Autodesk Fusion 360 part; units mm, degrees
sketch "Sketch1" plane through (0, 0, 0) normal (0, 0, 1) x (1, 0, 0)
  circle A0 centre (0, 0) radius 44.45
  arc A1 (38.1661, 38.1661) -> (-38.1661, 38.1661) centre (0, 0) ccw
  line L0 (0, 0) -> (38.1661, 38.1661) construction
  line L1 (0, 0) -> (-38.1661, 38.1661) construction
  line L2 (-38.1661, 38.1661) -> (-31.4309, 31.4309) construction
  line L3 (-38.1661, 38.1661) -> (-31.4309, 31.4309)
  line L4 (31.4309, 31.4309) -> (38.1661, 38.1661)
  line L5 (0, 0) -> (0, 53.975) construction
  line L6 (0, 53.975) -> (-31.4309, 31.4309) construction
  line L7 (0, 53.975) -> (31.4309, 31.4309) construction
  line L8 (-13.335, 80.645) -> (13.335, 80.645)
  line L9 (13.335, 80.645) -> (13.335, 53.975)
  line L10 (13.335, 53.975) -> (-13.335, 53.975) construction
  line L11 (-13.335, 53.975) -> (-13.335, 80.645)
  line L12 (-13.335, 53.975) -> (-13.335, 52.3018)
  line L13 (13.335, 53.975) -> (13.335, 52.3018)
  line L14 (-13.335, 67.31) -> (13.335, 67.31) construction
  circle A2 centre (0, 67.31) radius 11.049
  point P0 (-31.4309, 31.4309)
  point P1 (-13.335, 52.3018)
  point P2 (13.335, 52.3018)
  point P3 (-13.335, 67.31)
  point P4 (13.335, 67.31)
  dimension "d1" = 88.9
  dimension "d2" = 90
  dimension "d3" = 9.525
  dimension "d6" = 26.67
  dimension "d7" = 26.67
  dimension "d8" = 22.098
extrude "Extrude2" add sketch "Sketch1" along normal blind 50.8 contours A0 A1 L3 L4 | A1 L8 L9 L11 L12 L13
fillet "Fillet1" radius 5 2 edges at (-38.1661, 38.1661, 25.4) (38.1661, 38.1661, 25.4)
fillet "Fillet2" radius 15 2 edges at (-13.335, 52.3018, 25.4) (13.335, 52.3018, 25.4)
fillet "Fillet3" radius 5 2 edges at (-13.335, 80.645, 25.4) (13.335, 80.645, 25.4)
sketch "Sketch4" plane through (0, 80.645, 0) normal (0, 1, 0) x (-1, 0, 0)
  line L0 (-8.335, 50.8) -> (-8.335, 0)
  line L1 (-8.335, 0) -> (8.335, 0)
  line L2 (8.335, 0) -> (8.335, 50.8)
  line L3 (8.335, 50.8) -> (-8.335, 50.8)
  line L4 (0, 0) -> (0, 16.9333) construction
  line L5 (0, 16.9333) -> (0, 33.8667) construction
  line L6 (0, 33.8667) -> (0, 50.8) construction
  circle A0 centre (0, 16.9333) radius 1.778
  circle A1 centre (0, 33.8667) radius 1.778
  dimension "d17" = 3.556
  dimension "d18" = 3.556
extrude "Extrude3" cut sketch "Sketch4" along normal up to surface contours A0 | A1 end surface at (10.9941, 66.2099, 33.8667)
sketch "Sketch6" plane through (0, 0, 50.8) normal (0, 0, 1) x (-1, 0, 0)
  arc A0 (-13.335, -75.645) -> (-8.335, -80.645) centre (-8.335, -75.645) ccw
  line L0 (-8.335, -80.645) -> (8.335, -80.645)
  arc A1 (8.335, -80.645) -> (13.335, -75.645) centre (8.335, -75.645) ccw
  line L1 (13.335, -75.645) -> (13.335, -62.8862)
  arc A2 (22.173, -49.2104) -> (13.335, -62.8862) centre (28.335, -62.8862) ccw
  arc A3 (22.173, -49.2104) -> (34.0702, -41.8632) centre (0, 0) ccw
  arc A4 (34.0702, -41.8632) -> (34.4496, -34.4496) centre (30.9141, -37.9851) ccw
  line L2 (34.4496, -34.4496) -> (31.4309, -31.4309)
  arc A5 (-31.4309, -31.4309) -> (31.4309, -31.4309) centre (0, 0) ccw
  line L3 (-31.4309, -31.4309) -> (-34.4496, -34.4496)
  arc A6 (-34.4496, -34.4496) -> (-34.0702, -41.8632) centre (-30.9141, -37.9851) ccw
  arc A7 (-34.0702, -41.8632) -> (-22.173, -49.2104) centre (0, 0) ccw
  arc A8 (-13.335, -62.8862) -> (-22.173, -49.2104) centre (-28.335, -62.8862) ccw
  line L4 (-13.335, -62.8862) -> (-13.335, -75.645)
  circle A9 centre (0, -67.31) radius 11.049
  line L5 (0, -56.261) -> (0, -44.45)
  circle A10 centre (0, -67.31) radius 11.049
  circle A11 centre (0, 0) radius 44.45
  line L6 (0.25, -56.261) -> (-0.25, -56.261)
  line L7 (-0.25, -56.261) -> (-0.25, -44.45)
  line L8 (-0.25, -44.45) -> (0.25, -44.45)
  line L9 (0.25, -44.45) -> (0.25, -56.261)
  line L10 (0, 0) -> (0, -53.975)
  dimension "d22" = 0.5
extrude "Extrude4" cut sketch "Sketch6" against normal blind 0.5 contours A5 L5 A11 L6 L7 L8 L10 | A5 L5 A11 L6 L8 L9 L10
Could you check a few things on this model? Use its own coordinates, in mm. A direction names the side the tool comes from. Give positions to 0.01 mm unless a question says otherwise; leave off trailing zeros. Loops run counter-clockwise (first coordinate to the right, second up) from the corner with the lowest first, then second, coordinate; pieces in that order, holes last. Notation, with made-up numbers: (87.5, 19.25) -> (145.5, 19.25) arc R12 ccw to (145.5, 30.25) -> close; hole circle Ø5 at (-21, 46). An arc over 180 degrees is marked (long way). Return JSON: item names as keys, results as strings.
Item 1: If we section it at B-B on z = 28.5: List the corners of the cut face in (x, y) for me (3 decimals), plus the area to 3 significant figures.
Geometry results:
{"outline": "(-34.45, 34.45) -> (-31.431, 31.431) arc R44.45 cw to (31.431, 31.431) -> (34.45, 34.45) arc R5 ccw to (34.07, 41.863) arc R53.975 ccw to (22.173, 49.21) arc R15 cw to (13.335, 62.886) -> (13.335, 75.645) arc R5 ccw to (8.335, 80.645) -> (-8.335, 80.645) arc R5 ccw to (-13.335, 75.645) -> (-13.335, 62.886) arc R15 cw to (-22.173, 49.21) arc R53.975 ccw to (-34.07, 41.863) arc R5 ccw to start; hole circle Ø22.098 at (0, 67.31)", "area": "1,090 mm²"}
Item 2: If we section it at C-C on x = -6: List the corners of the cut face in (y, z) for me (3 decimals).
Geometry results:
{"outline": "(44.043, 0) -> (58.032, 0) -> (58.032, 50.8) -> (44.043, 50.8) -> close; (76.588, 0) -> (80.645, 0) -> (80.645, 50.8) -> (76.588, 50.8) -> close"}
Item 3: Which directions (+Z, -Z, +X, -X, +Y, -Y) give clear straight access to the entire face, cutting with the end or side of a thin tool? Please do faces 4 (the flat face through (0, 80.645, 25)), 5 (the flat face through (13.335, 69, 25)), 6 (the cylindrical face through (0.23, 79.45, 35.63)), 7 (the flat face through (-13.335, 69, 25)).
Geometry results:
{"face 4": "+Z, -Z, +X, -X, +Y", "face 5": "+Z, -Z, +X, +Y", "face 6": "+Y", "face 7": "+Z, -Z, -X, +Y"}
Item 4: We'd pull the mould along X, two halves only. Please class faces 1 (the flat face through (0, 51, 0)), 2 (the cylindrical face through (-0.489, 44.447, 25.044)), 3 (the cylindrical face through (28.277, 45.975, 25.044)): +X half, -X half, draft (parallel to the pull), parting line (faces both ways), or undercut.
Geometry results:
{"face 1": "draft", "face 2": "undercut", "face 3": "+X half"}
Item 5: I need wall thicknesses on L1, parallel to Z at x = 0, y = 79.85; L2, parallel to X at y = 67, z = 25 (3 decimals); L3, parallel to Y at x = 0, z = 23 (3 decimals). Which ranges of each line are inside material? Lowest first, please. Write a range as from..to.
Geometry results:
{"L1": "z = 0..15.16, 18.71..32.09, 35.64..50.8", "L2": "x = -13.335..-11.045, 11.045..13.335", "L3": "y = 44.45..56.261, 78.359..80.645"}
Item 6: If we section it at D-D on x = 24.5: List the corners of the cut face in (y, z) for me.
Geometry results:
{"outline": "(37.09, 0) -> (48.09, 0) -> (48.09, 50.8) -> (37.09, 50.8) -> close"}
Item 7: If we section it at A-A on y = 67.31: List the corners of the cut face in (x, z) for me (3 decimals), plus the area to 3 significant figures.
Geometry results:
{"outline": "(-13.335, 0) -> (-11.049, 0) -> (-11.049, 50.8) -> (-13.335, 50.8) -> close; (11.049, 0) -> (13.335, 0) -> (13.335, 50.8) -> (11.049, 50.8) -> close", "area": "232 mm²"}
Item 8: I'm going to push flat-ended pins straight in: pin 1 (2 mm diameter, centred on x = 24.5, z = 17, fed in from -Y); pin 2 (5 mm diameter, centred on x = 15, z = 16, fed in from -Y); pin 3 (0.6 mm diameter, centred on y = 50.5, z = 50.5, fed in from +X). Where does each tip first touch, or does it pass through?
Geometry results:
{"pin 1": "stops at y = 36.41", "pin 2": "stops at y = 40.86", "pin 3": "stops at x = 20.33"}
